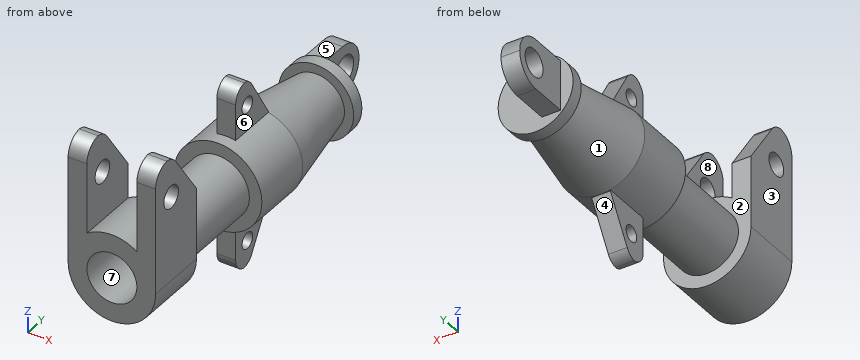
```python
from build123d import *

# Parameters (mm, degrees)
SKETCH1_R           = 35
BOSS_EXTRUDE1_DEPTH = 50
SKETCH6_R           = 25
BOSS_EXTRUDE2_DEPTH = 80
SKETCH7_R           = 35
BOSS_EXTRUDE3_DEPTH = 50
SKETCH10_R          = 30
BOSS_EXTRUDE5_DEPTH = 10
SKETCH12_W          = 70
SKETCH12_H          = 100.009163948
BOSS_EXTRUDE6_DEPTH = 50
CUT_EXTRUDE1_DEPTH  = 288.231322933
CUT_EXTRUDE2_DEPTH  = 281.761166962
FILLET1_R           = 15
SKETCH15_R          = 9
CUT_EXTRUDE3_DEPTH  = 288.208392811
BOSS_EXTRUDE8_DEPTH = 7.5
FILLET2_R           = 12
SKETCH17_R          = 6.5
CUT_EXTRUDE4_DEPTH  = 282.771025659
FILLET3_R           = 12
SKETCH18_W          = 15
SKETCH18_H          = 40
BOSS_EXTRUDE9_DEPTH = 50
CUT_EXTRUDE5_DEPTH  = 331.323570005
SKETCH20_R          = 11
CUT_EXTRUDE6_DEPTH  = 331.323570005
SKETCH21_R          = 20
CUT_EXTRUDE7_DEPTH  = 235


with BuildPart() as part:
    # Sketch1 → Boss-Extrude1 (new body)
    with BuildSketch(Plane(origin=(0, 0, 0), x_dir=(1, 0, 0), z_dir=(0, 1, 0))):
        with Locations(Location((0, 0, 0), (0, 0, 270))):
            Circle(SKETCH1_R)
    extrude(amount=BOSS_EXTRUDE1_DEPTH)

    # Sketch6 → Boss-Extrude2 (add)
    with BuildSketch(Plane(origin=(0, 50, 0), x_dir=(1, 0, 0), z_dir=(0, 1, 0))):
        with Locations(Location((0, 0, 0), (0, 0, 270))):
            Circle(SKETCH6_R)
    extrude(amount=BOSS_EXTRUDE2_DEPTH)

    # Sketch7 → Boss-Extrude3 (add)
    with BuildSketch(Plane(origin=(0, 130, 0), x_dir=(1, 0, 0), z_dir=(0, 1, 0))):
        with Locations(Location((0, 0, 0), (0, 0, 270))):
            Circle(SKETCH7_R)
    extrude(amount=BOSS_EXTRUDE3_DEPTH)



with BuildPart() as body_2:
    # Sketch10 → Boss-Extrude5 (new body)
    with BuildSketch(Plane(origin=(0, 250, 0), x_dir=(1, 0, 0), z_dir=(0, 1, 0))):
        with Locations(Location((0, 0, 0), (0, 0, 270))):
            Circle(SKETCH10_R)
    extrude(amount=BOSS_EXTRUDE5_DEPTH)


with BuildPart() as part_1:
    add(part.part)

    add(body_2.part)  # Revolve1 merges body 2
    # Sketch11 → Revolve1 (revolve)
    with BuildSketch(Plane(origin=(0, 0, 0), x_dir=(0, 0, -1), z_dir=(1, 0, 0))):
        Polygon((0, 250), (22.65711135, 250), (35, 180), (0, 180), align=None)
    revolve(axis=Axis((0, 180, 0), (0, 1, 0)))

    # Sketch12 → Boss-Extrude6 (add)
    with BuildSketch(Plane.XZ):
        with Locations((0, 50.004581974)):
            Rectangle(SKETCH12_W, SKETCH12_H)
    extrude(amount=-BOSS_EXTRUDE6_DEPTH)

    # Sketch13 → Cut-Extrude1 (cut, through all)
    with BuildSketch(Plane.ZY.offset(35)):
        Polygon((57.164723746, 50), (100.009163948, 20), (100.009163948, 50), align=None)
    extrude(amount=-CUT_EXTRUDE1_DEPTH, mode=Mode.SUBTRACT)

    # Sketch14 → Cut-Extrude2 (cut, through all)
    with BuildSketch(Plane.XZ):
        with BuildLine():
            Line((-20, 108.740570097), (20, 108.740570097))
            Line((20, 108.740570097), (20, 28.722813233))
            ThreePointArc((20, 28.722813233), (0, 35), (-20, 28.722813233))
            Line((-20, 28.722813233), (-20, 108.740570097))
        make_face()
    extrude(amount=-CUT_EXTRUDE2_DEPTH, mode=Mode.SUBTRACT)

    # Fillet1
    # the kernel refuses this fillet: 15 mm, written as the material it takes off along each edge
    with BuildSketch(Plane(origin=(-17.5, 0, 100.009163948), x_dir=(0, 0, -1), z_dir=(1, 0, 0)), Plane(origin=(-72.5, 0, 100.009163948), x_dir=(0, 0, -1), z_dir=(1, 0, 0))) as fillet1_piece_1:
        with BuildLine():
            CenterArc((FILLET1_R, FILLET1_R), FILLET1_R, 180, 90)
            Line((0, FILLET1_R), (0, 0))
            Line((0, 0), (FILLET1_R, 0))
        make_face()
    extrude(amount=90, mode=Mode.SUBTRACT)
    with BuildSketch(Plane(origin=(0.478735604, 20, 100.009163948), x_dir=(0, -1, 0), z_dir=(1, 0, 0)), Plane(origin=(-54.521264396, 20, 100.009163948), x_dir=(0, -1, 0), z_dir=(1, 0, 0))) as fillet1_piece_2:
        with BuildLine():
            CenterArc((FILLET1_R * 0.520567050552, FILLET1_R), FILLET1_R, 215, 55)
            Line((-FILLET1_R * 0.298584993737, FILLET1_R * 0.426423563649), (0, 0))
            Line((0, 0), (FILLET1_R * 0.520567050552, 0))
        make_face()
    extrude(amount=54.042528791, mode=Mode.SUBTRACT)

    # Sketch15 → Cut-Extrude3 (cut, through all)
    with BuildSketch(Plane.ZY.offset(35)):
        with Locations((67.943288424, 19)):
            Circle(SKETCH15_R)
    extrude(amount=-CUT_EXTRUDE3_DEPTH, mode=Mode.SUBTRACT)

    # Sketch16 → Boss-Extrude8 (add, symmetric)
    with BuildSketch(Plane(origin=(0, 0, 0), x_dir=(0, 0, -1), z_dir=(1, 0, 0))):
        Polygon((-35, 180), (-75, 155.965575239), (-75, 140), (-35, 140), (0, 140), (0, 180), align=None)
    boss_extrude8 = extrude(amount=BOSS_EXTRUDE8_DEPTH, both=True)

    # Fillet2
    # the kernel refuses this fillet: 12 mm, written as the material it takes off along each edge
    with BuildSketch(Plane(origin=(-37.5, 140, 75), x_dir=(0, 0, -1), z_dir=(1, 0, 0))) as fillet2_piece_1:
        with BuildLine():
            CenterArc((FILLET2_R, FILLET2_R), FILLET2_R, 180, 90)
            Line((0, FILLET2_R), (0, 0))
            Line((0, 0), (FILLET2_R, 0))
        make_face()
    extrude(amount=75, mode=Mode.SUBTRACT)
    with BuildSketch(Plane(origin=(-24.473183346, 155.965575239, 75), x_dir=(0, 0.5150380749100483, -0.8571673007021159), z_dir=(1, 0, 0))) as fillet2_piece_2:
        with BuildLine():
            CenterArc((FILLET2_R * 0.565772778188, -FILLET2_R), FILLET2_R, 90, 59)
            Line((-FILLET2_R * 0.291394522514, -FILLET2_R * 0.48496192509), (0, 0))
            Line((0, 0), (FILLET2_R * 0.565772778188, 0))
        make_face()
    extrude(amount=48.946366691, mode=Mode.SUBTRACT)

    # Sketch17 → Cut-Extrude4 (cut, through all)
    with BuildSketch(Plane(origin=(7.5, 0, 0), x_dir=(0, 0, -1), z_dir=(1, 0, 0))):
        with Locations((-55, 154.29)):
            Circle(SKETCH17_R)
    cut_extrude4 = extrude(amount=-CUT_EXTRUDE4_DEPTH, mode=Mode.SUBTRACT)

    # Mirror1: Boss-Extrude8 across plane
    add(boss_extrude8.mirror(Plane.XY))

    # Fillet3
    # the kernel refuses this fillet: 12 mm, written as the material it takes off along each edge
    with BuildSketch(Plane(origin=(-37.5, 140, -75), x_dir=(0, 0, 1), z_dir=(1, 0, 0))) as fillet3_piece_1:
        with BuildLine():
            CenterArc((FILLET3_R, -FILLET3_R), FILLET3_R, 90, 90)
            Line((0, -FILLET3_R), (0, 0))
            Line((0, 0), (FILLET3_R, 0))
        make_face()
    extrude(amount=75, mode=Mode.SUBTRACT)
    with BuildSketch(Plane(origin=(-24.473183346, 155.965575239, -75), x_dir=(0, 0.5150380749100483, 0.8571673007021159), z_dir=(1, 0, 0))) as fillet3_piece_2:
        with BuildLine():
            CenterArc((FILLET3_R * 0.565772778188, FILLET3_R), FILLET3_R, 211, 59)
            Line((-FILLET3_R * 0.291394522514, FILLET3_R * 0.48496192509), (0, 0))
            Line((0, 0), (FILLET3_R * 0.565772778188, 0))
        make_face()
    extrude(amount=48.946366691, mode=Mode.SUBTRACT)

    # Mirror2: Cut-Extrude4 across plane
    add(cut_extrude4.mirror(Plane.XY), mode=Mode.SUBTRACT)

    # Sketch18 → Boss-Extrude9 (add)
    with BuildSketch(Plane(origin=(0, 260, 0), x_dir=(1, 0, 0), z_dir=(0, 1, 0))):
        with Locations((-12.5, 0)):
            Rectangle(SKETCH18_W, SKETCH18_H)
    extrude(amount=BOSS_EXTRUDE9_DEPTH)

    # Sketch19 → Cut-Extrude5 (cut, through all)
    with BuildSketch(Plane.ZY.offset(20)):
        with BuildLine():
            Line((20, 310), (-1.45e-07, 310))
            ThreePointArc((-1.45e-07, 310), (14.142135572, 304.142135675), (20, 290))
            Line((20, 290), (20, 310))
        make_face()
        with BuildLine():
            Line((-20, 310), (-20, 290))
            ThreePointArc((-20, 290), (-14.142135675, 304.142135572), (-1.45e-07, 310))
            Line((-1.45e-07, 310), (-20, 310))
        make_face()
    extrude(amount=-CUT_EXTRUDE5_DEPTH, mode=Mode.SUBTRACT)

    # Sketch20 → Cut-Extrude6 (cut, through all)
    with BuildSketch(Plane.ZY.offset(20)):
        with Locations((0, 292.448780647)):
            Circle(SKETCH20_R)
    extrude(amount=-CUT_EXTRUDE6_DEPTH, mode=Mode.SUBTRACT)

    # Sketch21 → Cut-Extrude7 (cut)
    with BuildSketch(Plane.XZ):
        with Locations(Location((0, 0, 0), (0, 0, 270))):
            Circle(SKETCH21_R)
    extrude(amount=-CUT_EXTRUDE7_DEPTH, mode=Mode.SUBTRACT)


solid = part_1.part
```
Source: CAD feature listing. Evaluate the final solid. Frame: model axes, mm. Face numbers are marked on the shaded views. A direction names the side the tool comes from. Coordinates: 2 decimals unless noted, no trailing zeros. Loops run counter-clockwise (first coordinate to the right, second up) from the corner with the lowest first, then second, coordinate; pieces in that order, holes last. Notation, with made-up numbers: M 1.5,67 L 48.5,67 A16 cw 48.5,90 Z; hole C 57.25,42.5 d4. An arc over 180 degrees is marked long. Use a Markdown table: item, result. Add a question column.
Q1. Draft query along Y for the marked faces 1, 2, 3 and 4. Return one class per face: pulls with the +Y half, pulls with the -Y half, needs draft (parallel to the pull), parting line crosses it, or undercut.
Q2. Section query C-C, the plane y = 19. Return loops of the section in (x, z), and give its area (3 significant figures).
Q3. Section query B-B, the plane z = 42.5. Return loops of the section in (x, y), and give its area (3 significant figures).
Q4. First-contact query: pin 1 (20 mm diameter, centred on y = 158, z = 51, fed in from -X); pin 2 (1 mm diameter, centred on x = 8.5, z = -55.5, fed in from +Y); pin 3 (3 mm diameter, centred on x = -21.5, y = 207.5, fed in from +Z); pin 4 (1.5 mm diameter, centred on x = 10.5, y = 48, fed in from +Z). Flat tips, straight axial feed; report the tip coordinate or a pass-through.
Q5. Section query D-D, the plane y = 89.5. Return loops of the section in (x, z), and give its area (3 significant figures).
Q6. Material intervals for L1, parallel to Y at x = -14, z = 0; L2, parallel to X at y = 45.5, z = 54.5; L3, parallel to Z at x = -1, y = 154, sorted ascending.
Q7. Section query A-A, the plane y = 154.29. Return loops of the section in (x, z).
Q8. Access query for the marked faces 5, 6, 7 and 8. Directions: +Z, -Z, +X, -X, +Y, -Y. A direction counts if a zero-diameter tool reaches every point of the face in a straight line with its end or side. Return the directions, or none.
Result:
| question | item | result |
|---|---|---|
| 1 | face 1 | undercut |
| 1 | face 2 | undercut |
| 1 | face 3 | needs draft |
| 1 | face 4 | pulls with the +Y half |
| 2 | outline | M -35,0 A35 ccw 35,0 L 35,58.94 L 20,58.94 L 20,28.72 A35 ccw -20,28.72 L -20,58.94 L -35,58.94 Z; M -35,76.94 L -20,76.94 L -20,98.37 L -35,98.37 Z; M 20,76.94 L 35,76.94 L 35,98.37 L 20,98.37 Z; hole C 0,0 d40 |
| 2 | area | 4,400 mm2 |
| 3 | outline | M -35,0 L -20,0 L -20,50 L -35,50 Z; M -7.5,140 L 7.5,140 L 7.5,175.49 L -7.5,175.49 Z; M 20,0 L 35,0 L 35,50 L 20,50 Z |
| 3 | area | 2,030 mm2 |
| 4 | pin 1 | stops at x = -7.5 |
| 4 | pin 2 | passes through |
| 4 | pin 3 | stops at z = 22.61 |
| 4 | pin 4 | stops at z = 33.61 |
| 5 | outline | C 0,0 d50; hole C 0,0 d40 |
| 5 | area | 707 mm2 |
| 6 | L1 | y = 235 to 281.45, 303.45 to 310 |
| 6 | L2 | x = -35 to -20, 20 to 35 |
| 6 | L3 | z = -73.99 to -61.49, -48.51 to -19.97, 19.97 to 48.51, 61.49 to 73.99 |
| 7 | outline | M -7.5,-73.86 L 7.5,-73.86 L 7.5,-61.5 L -7.5,-61.5 Z; M -7.5,-48.5 L 7.5,-48.5 L 7.5,-34.19 A35 ccw 7.5,34.19 L 7.5,48.5 L -7.5,48.5 L -7.5,34.19 A35 ccw -7.5,-34.19 Z; M -7.5,61.5 L 7.5,61.5 L 7.5,73.86 L -7.5,73.86 Z; hole C 0,0 d40 |
| 8 | face 5 | +Z, +X, -X, +Y |
| 8 | face 6 | +Z, +X, +Y, -Y |
| 8 | face 7 | -Y |
| 8 | face 8 | +Z, +Y, -Y |
